Verification items for the finished model (mm, model axes). Face numbers are marked on the shaded views. A direction names the side the tool comes from. Round coordinates to 2 decimals unless told otherwise and drop trailing zeros. Write each loop counter-clockwise with the first axis right and the second up, starting at its lowest first coordinate (ties: lowest second). Pieces come first, ordered by that corner, then holes. Notation, with made-up numbers: (6.25, -37.5) -> (23.25, -37.5) arc R19 cw to (23.25, -8.5) -> close; hole circle Ø10 at (39.5, 0.25). An arc over 180 degrees is marked (long way). Use CSV: the item, a comma, the result in double quotes.
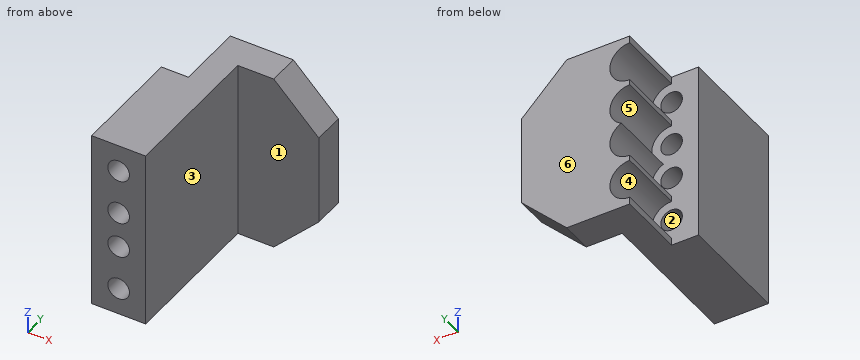
Autodesk Inventor part; units mm, degrees
ref_plane "YZ Plane" through (0, 0, 0) normal (1, 0, 0) x (0, 1, 0)
ref_plane "XZ Plane" through (0, 0, 0) normal (0, 1, 0) x (-1, 0, 0)
ref_plane "XY Plane" through (0, 0, 0) normal (0, 0, 1) x (1, 0, 0)
sketch "Sketch1" plane through (0, 0, 0) normal (0, 0, 1) x (1, 0, 0)
  line L0 (-7.5, 10) -> (7.5, 10)
  line L1 (7.5, 10) -> (7.5, -10)
  line L2 (7.5, -10) -> (-7.5, -10)
  line L3 (-7.5, -10) -> (-7.5, 10)
  point P0 (0, 0)
  dimension "d0" = 15
  dimension "d1" = 20
  dimension "d2" = 7.5
  dimension "d3" = 10
extrude "Extrusion1" add sketch "Sketch1" along normal blind 20
sketch "Sketch2" plane through (7.5, -10, 0) normal (1, 0, 0) x (0, 0, -1)
  line L0 (0, 20) -> (0, 0)
  line L1 (0, 20) -> (-20, 20)
  line L2 (-20, 0) -> (-20, 20)
  line L3 (0, 0) -> (-20, 0)
  line L4 (-20, 0) -> (0, 0)
  line L5 (0, 0) -> (0, 16.5)
  line L6 (0, 16.5) -> (-20, 16.5)
  line L7 (-20, 16.5) -> (-20, 0)
  point P0 (0, 10)
  dimension "d6" = 16.5
extrude "Extrusion2" cut sketch "Sketch2" against normal blind 9 contours L0 L3 L2 L6
sketch "Sketch3" plane through (-7.5, 10, 0) normal (0, 1, 0) x (1, 0, 0)
  circle A0 centre (3, -12) radius 0.7835
  circle A1 centre (3, -17) radius 0.7835
  line L0 (0, 0) -> (15, 0)
  line L1 (0, 0) -> (0, -20)
  line L2 (15, -20) -> (0, -20)
  line L3 (15, 0) -> (15, -20)
  circle A2 centre (3, -8) radius 0.7835
  circle A3 centre (3, -3) radius 0.7835
  point P0 (7.5, 0)
  dimension "d22" = 3
  dimension "d23" = 3
  dimension "d24" = 3
  dimension "d25" = 8
  dimension "d26" = 3
  dimension "d27" = 8
  dimension "d28" = 3
  dimension "d29" = 3
hole "Hole1" at (-4.5, 10, 12) at (-4.5, 10, 17) at (-4.5, 10, 8) at (-4.5, 10, 3) direction (0, -1, 0) diameter 2.4 end through all counterbore diameter 4.4 counterbore depth 7.5
sketch "Sketch4" plane through (-7.5, 10, 0) normal (0, 1, 0) x (1, 0, 0)
  arc A0 (2.0835, -10) -> (3.9165, -10) centre (3, -12) ccw
  circle A1 centre (3, -17) radius 2.2
  line L0 (0, 0) -> (15, 0)
  line L1 (0, 0) -> (0, -20)
  line L2 (15, -20) -> (0, -20)
  line L3 (15, 0) -> (15, -20)
  line L4 (15, 0) -> (10, 0)
  line L5 (10, 0) -> (15, -5)
  line L6 (15, 0) -> (15, -5)
  line L7 (15, -20) -> (15, -15)
  line L8 (15, -20) -> (10, -20)
  line L9 (10, -20) -> (15, -15)
  arc A2 (3.9165, -10) -> (2.0835, -10) centre (3, -8) ccw
  point P0 (7.5, 0)
  dimension "d16" = 5
  dimension "d17" = 5
  dimension "d18" = 5
  dimension "d19" = 5
extrude "Extrusion3" cut sketch "Sketch4" against normal through all contours L0 L3 L5 | L9 L3 L2
sketch "Sketch5" plane through (-7.5, 10, 20) normal (0, 1, 0) x (1, 0, 0)
  line L0 (15, 15) -> (10, 20)
  line L1 (0, 20) -> (10, 20)
  line L2 (0, 20) -> (0, 0)
  line L3 (10, 0) -> (0, 0)
  line L4 (10, 0) -> (15, 5)
  line L5 (15, 15) -> (15, 5)
  circle A0 centre (3, 17) radius 2.2
  circle A1 centre (3, 3) radius 2.2
  arc A2 (3.9165, 10) -> (2.0835, 10) centre (3, 12) ccw
  arc A3 (2.0835, 10) -> (3.9165, 10) centre (3, 8) ccw
  line L6 (0, 20) -> (3, 20)
  line L7 (3, 20) -> (3, 0)
  line L8 (3, 0) -> (0, 0)
  line L9 (0, 0) -> (0, 20)
  point P0 (7.5, 20)
  dimension "d30" = 3
extrude "Extrusion4" cut sketch "Sketch5" against normal blind 7.5 contours L7 A0 A2 A3 A1 L3 L2 L1 | L7 A0 | A1 L7 | L7 A3 A2 picked at (2.1729, 17.6329) picked at (2.3382, 2.4724) picked at (2.6945, 10)
properties part number "galvo_stop"
Q1. Section check D-D (x = 5). Record the cut outline in (y, z).
Filled in:
outline,"(6.5, 2.5) -> (10, 2.5) -> (10, 17.5) -> (6.5, 17.5) -> close"
Q2. Access from +Z, -Z, +X, -X, +Y, -Y to the whole of each face (thin tool, end or side, straight path). Record for the marked faces 5 and 6.
Filled in:
face 5,"-X, +Y"
face 6,"+Z, -Z, +X, -X, +Y"
Q3. Mould release check, pull along X, two halves, no side actions. Record for the marked faces 1, 2, 3 and 4: released by +X, released by -X, zero draft, split by the parting line, or undercut.
Filled in:
face 1,"zero draft"
face 2,"undercut"
face 3,"released by +X"
face 4,"released by -X"
Q4. Section check C-C (y = 4.5). Record the cut outline in (x, z).
Filled in:
outline,"(-4.5, 0) -> (-1.5, 0) -> (-1.5, 20) -> (-4.5, 20) -> (-4.5, 19.2) arc R2.2 cw to (-4.5, 14.8) -> (-4.5, 14.2) arc R2.2 cw to (-3.58, 10) arc R2.2 cw to (-4.5, 5.8) -> (-4.5, 5.2) arc R2.2 cw to (-4.5, 0.8) -> close"
Q5. Go/stop test with flat-tipped pins: P1, Ø1, axis at y = 4, z = 17, coming from the +X side; P2, Ø0.7, axis at y = 5, z = 5.5, coming from the -X side; P3, Ø3, axis at x = -4.5, z = 17, coming from the +Y side; P4, Ø1.4, axis at x = -4.5, z = 8, coming from the -Y side. Record where each tip stops, or that it passes through.
Filled in:
P1,"x = -1.5"
P2,"x = -4.5"
P3,"y = 2.5"
P4,"through"
Q6. Material ranges on L1, parallel to Z at x = -4.5, y = -3.25; L2, parallel to X at y = -0.5, z = 3; L3, parallel to Y at x = 3.5, z = 16.25, recorded low to high.
Filled in:
L1,"0 to 1.8, 4.2 to 6.8, 9.2 to 10.8, 13.2 to 15.8, 18.2 to 20"
L2,"-7.5 to -5.7, -3.3 to -1.5"
L3,"6.5 to 10"
Q7. Section check A-A (z = 3). Record the cut outline in (x, y).
Filled in:
outline,"(-7.5, -10) -> (-5.7, -10) -> (-5.7, 2.5) -> (-7.5, 2.5) -> close; (-3.3, -10) -> (-1.5, -10) -> (-1.5, 6.5) -> (5.5, 6.5) -> (5.5, 10) -> (-2.3, 10) -> (-2.3, 2.5) -> (-3.3, 2.5) -> close"
Q8. Section check B-B (z = 5.5). Record the cut outline in (x, y).
Filled in:
outline,"(-7.5, -10) -> (-1.5, -10) -> (-1.5, 6.5) -> (7.5, 6.5) -> (7.5, 10) -> (-4.5, 10) -> (-4.5, 2.5) -> (-7.5, 2.5) -> close"
